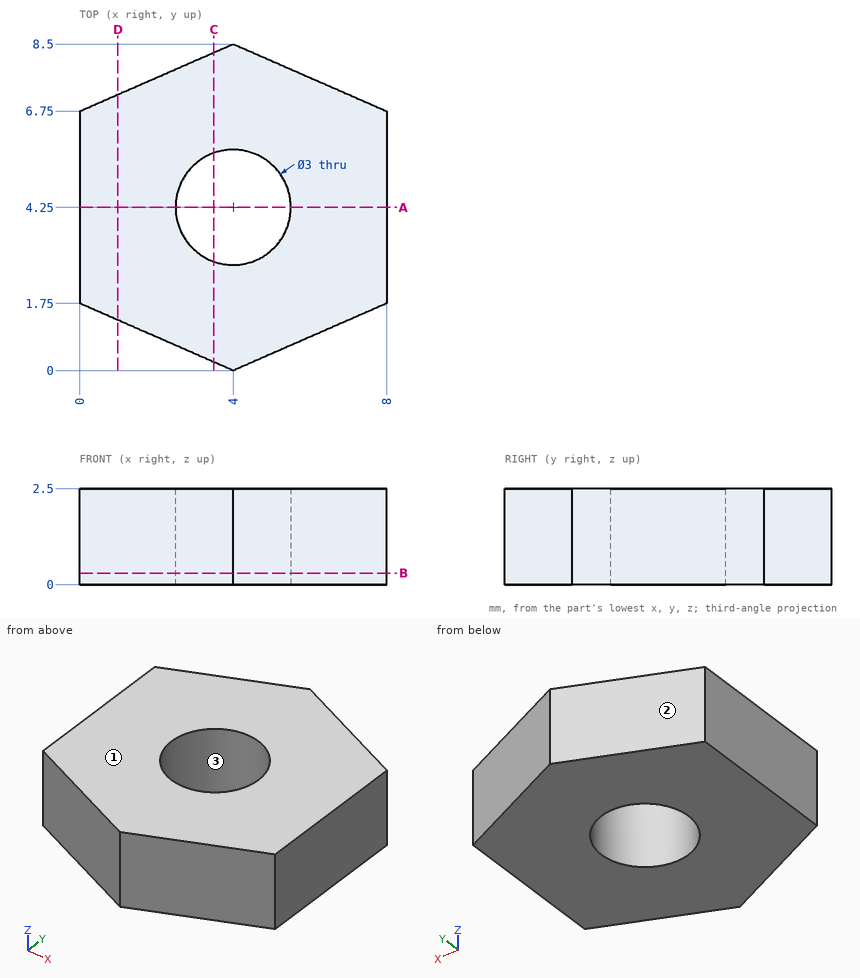
Geometry: see drawing. Coordinates: mm, zero at the bounding-box minimum. Round coordinates to 2 decimals unless told otherwise and drop trailing zeros. Loops run counter-clockwise (first coordinate to the right, second up) from the corner with the lowest first, then second, coordinate; pieces in that order, holes last. Notation, with made-up numbers: (28, 30.25) -> (85, 30.25) arc R33 cw to (85, 69.25) -> close; hole circle Ø1 at (3, 15.5). An arc over 180 degrees is marked (long way). One line per question, with ' | ' between items. Start each with the question number.
1. Section B-B on z = 0.3. Output: boundary loops of the cut face in (x, y), and give its area (3 significant figures).
2. Section C-C on x = 3.5. Output: boundary loops of the cut face in (y, z).
3. Section D-D on x = 1. Output: boundary loops of the cut face in (y, z), and give its area (3 significant figures).
4. Line query: line 1 along Y through (x, z) = (3.5, 1.7); line 2 along X through (y, z) = (4.75, 1.3); line 3 along Y through (x, z) = (3.25, 1.3). Output: solid intervals per line, ascending. Write a range as [from, to].
5. Mould query, pull axis Y, two halves, no side actions, for the marked faces 1, 2 and 3. Classes: pulls with the +Y half, pulls with the -Y half, needs draft (parallel to the pull), parting line crosses it, or undercut.
6. Section A-A on y = 4.25. Output: boundary loops of the cut face in (x, z).
Returned:
1) outline: (0, 1.75) -> (4, 0) -> (8, 1.75) -> (8, 6.75) -> (4, 8.5) -> (0, 6.75) -> close; hole circle Ø3 at (4, 4.25) | area: 46.9 mm2
2) outline: (0.22, 0) -> (2.84, 0) -> (2.84, 2.5) -> (0.22, 2.5) -> close; (5.66, 0) -> (8.28, 0) -> (8.28, 2.5) -> (5.66, 2.5) -> close
3) outline: (1.31, 0) -> (7.19, 0) -> (7.19, 2.5) -> (1.31, 2.5) -> close | area: 14.7 mm2
4) line 1: y = [0.22, 2.84], [5.66, 8.28] | line 2: x = [0, 2.59], [5.41, 8] | line 3: y = [0.33, 2.95], [5.55, 8.17]
5) face 1: needs draft | face 2: pulls with the +Y half | face 3: undercut
6) outline: (0, 0) -> (2.5, 0) -> (2.5, 2.5) -> (0, 2.5) -> close; (5.5, 0) -> (8, 0) -> (8, 2.5) -> (5.5, 2.5) -> close
